```python
from build123d import *

# Parameters (mm, degrees)
ESBO_O1_W                = 70.4
ESBO_O1_H                = 70.4
RESSALTO_EXTRUS_O1_DEPTH = 50


with BuildPart() as part:
    # Esboço1 → Ressalto-extrusão1 (new, symmetric)
    with BuildSketch(Plane.XY):
        with BuildLine():
            Line((-38, -40), (38, -40))
            ThreePointArc((38, -40), (39.414213562, -39.414213562), (40, -38))
            Line((40, -38), (40, 38))
            ThreePointArc((40, 38), (39.414213562, 39.414213562), (38, 40))
            Line((38, 40), (-38, 40))
            ThreePointArc((-38, 40), (-39.414213562, 39.414213562), (-40, 38))
            Line((-40, 38), (-40, -38))
            ThreePointArc((-40, -38), (-39.414213562, -39.414213562), (-38, -40))
        make_face()
        Rectangle(ESBO_O1_W, ESBO_O1_H, mode=Mode.SUBTRACT)
    extrude(amount=RESSALTO_EXTRUS_O1_DEPTH, both=True)


solid = part.part
```
The model under review builds one solid part; all positions refer to its coordinate system, in mm. A direction names the side the tool comes from. Round coordinates to 2 decimals unless told otherwise and drop trailing zeros. Loops run counter-clockwise (first coordinate to the right, second up) from the corner with the lowest first, then second, coordinate; pieces in that order, holes last. Notation, with made-up numbers: M 20,12.5 L 26,12.5 A23 ccw 26,30.5 Z; hole C -7,51 d11. An arc over 180 degrees is marked long. Answer as a JSON object with one key per item and string values.
(1) Take a section at B-B on z = -22. Give the boundary of the cut face in (x, y).
Resolved:
{"outline": "M -40,-38 A2 ccw -38,-40 L 38,-40 A2 ccw 40,-38 L 40,38 A2 ccw 38,40 L -38,40 A2 ccw -40,38 Z; hole M -35.2,-35.2 L 35.2,-35.2 L 35.2,35.2 L -35.2,35.2 Z"}
(2) Tool access review of faces 5 (the flat face through (0, 35.2, 1)), 6 (the flat face through (-1, -40, 1)): name each direction out of +Z, -Z, +X, -X, +Y, -Y from which nothing blocks a thin tool from reaching the whole face with its end or side.
Resolved:
{"face 5": "+Z, -Z", "face 6": "+Z, -Z, +X, -X, -Y"}
(3) Draft analysis for pull direction Y (two halves, no side actions). For faces 1 (the flat face through (40, -1, 1)), 2 (the flat face through (35.2, 0, 1)), 3 (the flat face through (0, -35.2, 1)), 4 (the flat face through (1, 40, 1)), state which applies: released by +Y, released by -Y, zero draft, split by the parting line, or undercut.
Resolved:
{"face 1": "zero draft", "face 2": "undercut", "face 3": "undercut", "face 4": "released by +Y"}
(4) To check wall thickness, follow line 1 along X through (y, z) = (-6.5, -4.5). State the ranges of the line that lie inside material, in increasing order.
Resolved:
{"line 1": "-40 to -35.2, 35.2 to 40"}
(5) Take a section at A-A on y = 17.5. Give the boundary of the cut face in (x, z), and give its area (3 significant figures).
Resolved:
{"outline": "M -40,-50 L -35.2,-50 L -35.2,50 L -40,50 Z; M 35.2,-50 L 40,-50 L 40,50 L 35.2,50 Z", "area": "960 mm²"}
